Autodesk Fusion 360 part; units mm, degrees
sketch "Szkic1" plane through (0, 0, 0) normal (0, 0, 1) x (1, 0, 0)
  line L0 (0, 0) -> (48, 0)
  line L1 (48, 0) -> (48, 81)
  line L2 (48, 81) -> (0, 81)
  line L3 (0, 81) -> (0, 0)
  dimension "d1" = 48
  dimension "d2" = 81
extrude "Wyciągnięcie proste1" add sketch "Szkic1" along normal blind 2 makes body 1
ref_plane "Płaszczyzna konstrukcyjna1" through (0, 0, 2) normal (0, 0, 1) x (1, 0, 0)
sketch "Szkic2" plane through (0, 0, 2) normal (0, 0, 1) x (1, 0, 0)
  line L0 (0, 2) -> (2, 2) construction
  line L1 (0, 0) -> (48, 0)
  line L2 (48, 0) -> (48, 81)
  line L3 (48, 81) -> (0, 81)
  line L4 (0, 81) -> (0, 0)
  line L5 (2, 2) -> (12, 2)
  line L6 (12, 2) -> (12, 0)
  line L7 (12, 0) -> (2, 0)
  line L8 (2, 0) -> (2, 2)
  line L9 (46, 2) -> (36, 2)
  line L10 (36, 2) -> (36, 0)
  line L11 (36, 0) -> (46, 0)
  line L12 (46, 0) -> (46, 2)
  line L13 (0, 0) -> (2, 0)
  line L14 (2, 0) -> (2, 81)
  line L15 (2, 81) -> (0, 81)
  line L16 (0, 81) -> (0, 0)
  line L17 (48, 0) -> (46, 0)
  line L18 (46, 0) -> (46, 81)
  line L19 (46, 81) -> (48, 81)
  line L20 (48, 81) -> (48, 0)
  dimension "d8" = 44
  dimension "d10" = 48
  dimension "d11" = 81
  dimension "d12" = 10
  dimension "d13" = 2
  dimension "d16" = 10
  dimension "d19" = 81
  dimension "d22" = 81
extrude "Wyciągnięcie proste2" add sketch "Szkic2" along normal blind 5 contours L1 L5 L6 L7 L8 L14 bodies 1
extrude "Wyciągnięcie proste3" add sketch "Szkic2" along normal blind 5 contours L1 L9 L10 L11 L12 L18 bodies 1
extrude "Wyciągnięcie proste4" add sketch "Szkic2" along normal blind 31 contours L1 L3 L4 L8 L13 L14 L15 L16 bodies 1
extrude "Wyciągnięcie proste5" add sketch "Szkic2" along normal blind 31 contours L1 L2 L3 L12 L17 L18 L19 L20 bodies 1
ref_plane "Płaszczyzna konstrukcyjna2" through (0, 0, 33) normal (0, 0, 1) x (1, 0, 0)
sketch "Szkic3" plane through (0, 0, 33) normal (0, 0, 1) x (1, 0, 0)
  line L0 (0, 0) -> (48, 0)
  line L1 (48, 0) -> (48, 81)
  line L2 (48, 81) -> (0, 81)
  line L3 (0, 81) -> (0, 0)
  dimension "d26" = 48
  dimension "d27" = 81
extrude "Wyciągnięcie proste6" add sketch "Szkic3" along normal blind 2 bodies 1
copy_body "Bryła->Komponent1" bodies 1 removing the originals makes body 2 in component "Component"
component "Component" placed x (1, 0, 0) y (0, 1, 0) z (0, 0, 1) at (0, 0, 0)
Build history of the part. All positions in model axes, mm. A direction names the side the tool comes from. Coordinates: 2 decimals unless noted, no trailing zeros. Write each loop counter-clockwise with the first axis right and the second up, starting at its lowest first coordinate (ties: lowest second). Pieces come first, ordered by that corner, then holes.
(1) Cut at A-A on z = 3. List the corners of the cut face in (x, y), and give its area (3 significant figures).
(2) Mould opens along Z. For faces 1 (the flat face through (24, 41, 35)), 2 (the flat face through (0, 41, 17)), 3 (the flat face through (12, 1, 4)) say: pulls with the +Z half, pulls with the -Z half, needs draft (parallel to the pull), parting line crosses it, or undercut.
(3) 3-axis set-ups, long thin cutter, end or side, ignore diameter. For faces 4 (the flat face through (48, 40, 17)), 5 (the flat face through (41, 1, 7)), 6 (the flat face through (46, 40, 17)): which of +Z, -Z, +X, -X, +Y, -Y reach the whole face in a straight line?
(4) Cut at C-C on y = 72.5. List the corners of the cut face in (x, z).
(5) Cut at B-B on x = 33. List the corners of the cut face in (y, z).
(6) Pin check, flat tips, straight feed: pin 1 Ø1.5 at (y, z) = (54, 29) entering from -X; pin 2 Ø1.5 at (x, z) = (7, 4) entering from +Y. Stop position of each tip, or through.
(7) Drill centre lines: line 1 (X direction, y = 41.5, z = 31.5); line 2 (Z direction, x = 40, y = 51); line 3 (Y direction, x = 9, z = 4). Where is each one in solid material? Low to high.
(8) Cut at D-D on z = 8. List the corners of the cut face in (x, y), and give its area (3 significant figures).
Working result:
1. outline: (0, 0) - (12, 0) - (12, 2) - (2, 2) - (2, 81) - (0, 81) - close; (36, 0) - (48, 0) - (48, 81) - (46, 81) - (46, 2) - (36, 2) - close
1. area: 364 mm2
2. face 1: pulls with the +Z half
2. face 2: needs draft
2. face 3: undercut
3. face 4: +Z, -Z, +X, +Y, -Y
3. face 5: +Y, -Y
3. face 6: +Y
4. outline: (0, 0) - (48, 0) - (48, 35) - (0, 35) - close; hole (2, 2) - (46, 2) - (46, 33) - (2, 33) - close
5. outline: (0, 0) - (81, 0) - (81, 2) - (0, 2) - close; (0, 33) - (81, 33) - (81, 35) - (0, 35) - close
6. pin 1: stops at x = 0
6. pin 2: stops at y = 2
7. line 1: x = 0 to 2, 46 to 48
7. line 2: z = 0 to 2, 33 to 35
7. line 3: y = 0 to 2
8. outline: (0, 0) - (2, 0) - (2, 81) - (0, 81) - close; (46, 0) - (48, 0) - (48, 81) - (46, 81) - close
8. area: 324 mm2
